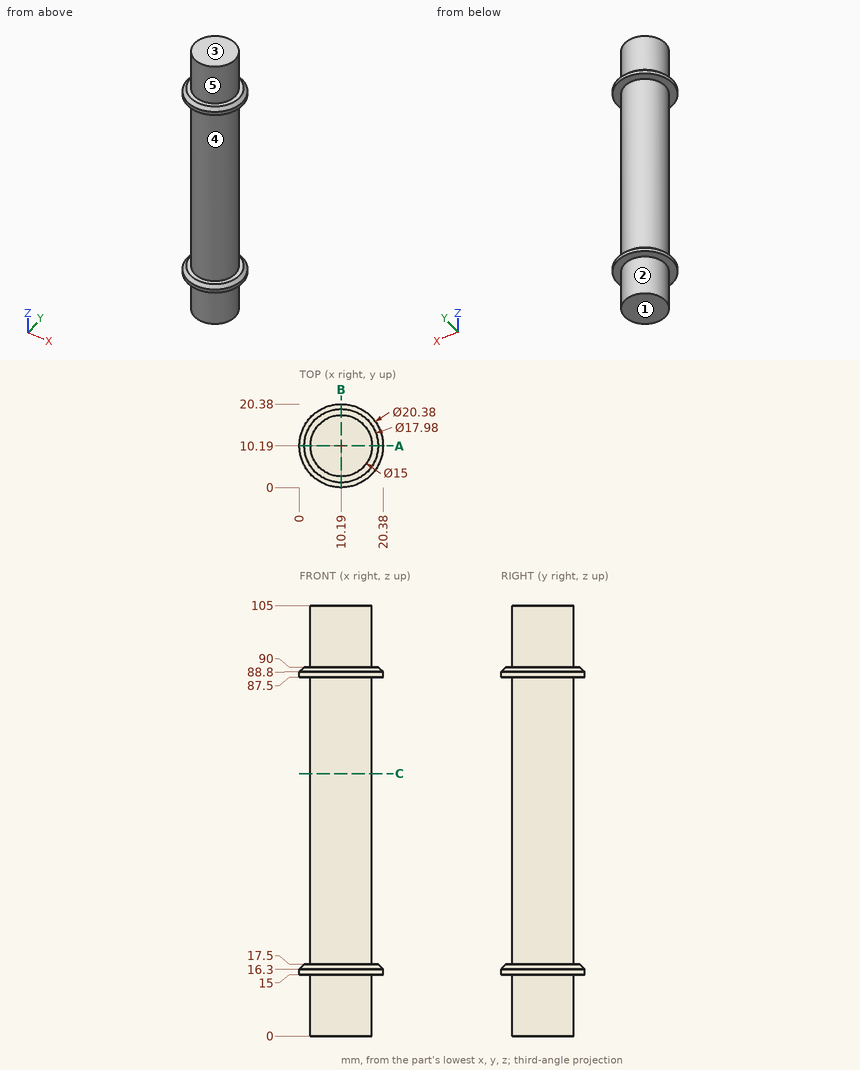
Geometry: see drawing. Coordinates: mm, zero at the bounding-box minimum. A direction names the side the tool comes from. Round coordinates to 2 decimals unless told otherwise and drop trailing zeros. Loops run counter-clockwise (first coordinate to the right, second up) from the corner with the lowest first, then second, coordinate; pieces in that order, holes last. Notation, with made-up numbers: M -29.5,-1 L 13.5,-1 A19 cw 13.5,36 Z; hole C -30,-13 d7. An arc over 180 degrees is marked long. Use a Markdown table: item, result. Add a question column.
1. Reachability of the marked faces 1 and 2 from +Z, -Z, +X, -X, +Y, -Y: full face, straight path, thin tool, end or side. Return the list, or none.
2. Contact query for flat-ended pins moving along their axis: P1, Ø1.5, axis at x = 13.5, z = 89, coming from the +Y side; P2, Ø1, axis at y = 11, z = 93.5, coming from the +X side; P3, Ø2, axis at x = 4.5, z = 81.5, coming from the -Y side; P4, Ø12, axis at x = 9, z = 89.5, coming from the -Y side. Output: stop coordinate, or through.
3. Line query: line 1 (Z direction, x = 10.5, y = 19); line 2 (X direction, y = 10, z = 10); line 3 (X direction, y = 4.75, z = 33). Output: solid intervals per line, ascending.
4. Mould query, pull axis Z, two halves, no side actions, for the marked faces 3, 4 and 5. Classes: pulls with the +Z half, pulls with the -Z half, needs draft (parallel to the pull), parting line crosses it, or undercut.
5. Section query A-A on y = 10.19. Return the cut outline in (x, z), then the cut area to 3 significant figures.
6. Section query C-C on z = 64. Return the cut outline in (x, y), then the cut area to 3 significant figures.
Reported:
| question | item | result |
|---|---|---|
| 1 | face 1 | -Z, +X, -X, +Y, -Y |
| 1 | face 2 | -Z |
| 2 | P1 | stops at y = 20.05 |
| 2 | P2 | stops at x = 17.68 |
| 2 | P3 | stops at y = 4.34 |
| 2 | P4 | stops at y = 0 |
| 3 | line 1 | z = 15 to 17.5, 87.5 to 90 |
| 3 | line 2 | x = 2.69 to 17.69 |
| 3 | line 3 | x = 5.03 to 15.35 |
| 4 | face 3 | pulls with the +Z half |
| 4 | face 4 | undercut |
| 4 | face 5 | needs draft |
| 5 | outline | M 0,15 L 2.69,15 L 2.69,0 L 17.69,0 L 17.69,15 L 20.38,15 L 20.38,16.3 L 19.18,17.5 L 17.69,17.5 L 17.69,87.5 L 20.38,87.5 L 20.38,88.8 L 19.18,90 L 17.69,90 L 17.69,105 L 2.69,105 L 2.69,90 L 1.2,90 L 0,88.8 L 0,87.5 L 2.69,87.5 L 2.69,17.5 L 1.2,17.5 L 0,16.3 Z |
| 5 | area | 1,600 mm² |
| 6 | outline | C 10.19,10.19 d15 |
| 6 | area | 177 mm² |
